Autodesk Inventor part; units mm, degrees
ref_plane "YZ Plane" through (0, 0, 0) normal (1, 0, 0) x (0, 1, 0)
ref_plane "XZ Plane" through (0, 0, 0) normal (0, 1, 0) x (-1, 0, 0)
ref_plane "XY Plane" through (0, 0, 0) normal (0, 0, 1) x (1, 0, 0)
sketch "Sketch1" plane through (0, 0, 0) normal (0, 1, 0) x (-1, 0, 0)
  line L0 (32.355, 4.45) -> (-32.355, 4.45)
  line L1 (-32.355, 4.45) -> (-32.355, -4.45)
  line L2 (-32.355, -4.45) -> (32.355, -4.45)
  line L3 (32.355, -4.45) -> (32.355, 4.45)
  point P0 (0, 0)
  dimension "d0" = 64.71
  dimension "d1" = 32.355
  dimension "d2" = 8.9
  dimension "d3" = 4.45
extrude "Extrusion1" add sketch "Sketch1" along normal blind 7.8
sketch "Sketch2" plane through (0, 0, 0) normal (0, 1, 0) x (-1, 0, 0)
  line L0 (-32.355, 4.45) -> (-32.355, -4.45)
  line L1 (-32.355, -3.45) -> (-37.945, -3.45)
  line L2 (-37.945, -3.45) -> (-37.945, 6.25)
  line L3 (-37.945, 6.25) -> (-32.355, 6.25)
  line L4 (-32.355, 6.25) -> (-32.355, -3.45)
  line L5 (-32.355, -4.45) -> (32.355, -4.45)
  line L6 (32.355, -4.45) -> (32.355, 4.45)
  line L7 (32.355, -3.45) -> (37.855, -3.45)
  line L8 (37.855, -3.45) -> (37.855, 6.25)
  line L9 (37.855, 6.25) -> (32.355, 6.25)
  line L10 (32.355, 6.25) -> (32.355, -3.45)
  point P0 (0, 0)
  dimension "d6" = 10.7
  dimension "d7" = 5.59
  dimension "d8" = 10.7
  dimension "d9" = 5.5
  dimension "d10" = 1
  dimension "d11" = 1
extrude "Extrusion2" add sketch "Sketch2" along normal blind 5
sketch "Sketch3" plane through (-32.355, 7.8, 4.45) normal (0, 0, 1) x (1, 0, 0)
  line L0 (0, -2.8) -> (0, 0)
  line L1 (64.71, -7.8) -> (64.71, 0)
  line L2 (0, -2.8) -> (64.71, -2.8)
  line L3 (64.71, -2.8) -> (64.71, -1.35)
  line L4 (64.71, -1.35) -> (0, -1.35)
  line L5 (0, -1.35) -> (0, -2.8)
  point P0 (32.355, -7.8)
  dimension "d14" = 1.45
extrude "Extrusion3" cut sketch "Sketch3" against normal blind 5
sketch "Sketch4" plane through (0, 5, 0) normal (0, 1, 0) x (1, 0, 0)
  line L0 (32.355, -6.25) -> (37.945, -6.25)
  line L1 (37.945, 3.45) -> (32.355, 3.45)
  line L2 (37.945, -6.25) -> (32.355, -6.25)
  line L3 (32.355, -6.25) -> (32.355, 3.45)
  line L4 (32.355, 3.45) -> (37.945, 3.45)
  line L5 (37.945, 3.45) -> (37.945, -6.25)
  line L6 (-37.855, -6.25) -> (-32.355, -6.25)
  line L7 (-32.355, 3.45) -> (-37.855, 3.45)
  line L8 (-37.855, -6.25) -> (-32.355, -6.25)
  line L9 (-32.355, -6.25) -> (-32.355, 3.45)
  line L10 (-32.355, 3.45) -> (-37.855, 3.45)
  line L11 (-37.855, 3.45) -> (-37.855, -6.25)
  line L12 (-37.355, -5.75) -> (-32.855, -5.75)
  line L13 (-32.855, -5.75) -> (-32.855, 2.95)
  line L14 (-32.855, 2.95) -> (-37.355, 2.95)
  line L15 (-37.355, 2.95) -> (-37.355, -5.75)
  line L16 (32.855, -5.75) -> (37.445, -5.75)
  line L17 (37.445, -5.75) -> (37.445, 2.95)
  line L18 (37.445, 2.95) -> (32.855, 2.95)
  line L19 (32.855, 2.95) -> (32.855, -5.75)
  point P0 (0, 0)
  dimension "d17" = 0.5
  dimension "d18" = 0.5
extrude "Extrusion4" add sketch "Sketch4" along normal blind 0.5 contours L15 L14 L13 L12 | L19 L18 L17 L16
sketch "Sketch5" plane through (0, 5.5, 0) normal (0, 1, 0) x (1, 0, 0)
  circle A0 centre (35.205, -4.05) radius 1.15
  circle A1 centre (-35.205, -4.1) radius 1.15
  point P0 (0, 0)
  dimension "d21" = 4.1
  dimension "d22" = 4.05
  dimension "d23" = 70.41
  dimension "d24" = 35.205
  dimension "d35" = 2.3
  dimension "d36" = 2.3
extrude "Extrusion5" cut sketch "Sketch5" against normal through all
sketch "Sketch6" plane through (0, 0, 0) normal (0, -1, 0) x (1, 0, 0)
  circle A0 centre (30.75, 0) radius 0.75
  circle A1 centre (-30.75, 0) radius 0.75
  point P0 (0, 0)
  dimension "d27" = 61.5
  dimension "d28" = 30.75
  dimension "d29" = 1.5
  dimension "d30" = 1.5
  dimension "d33" = 0
  dimension "d34" = 0
extrude "Extrusion6" add sketch "Sketch6" along normal blind 1
sketch "Sketch7" plane through (-32.355, 0, 4.45) normal (0, 0, 1) x (1, 0, 0)
  line L0 (64.71, 0) -> (0, 0)
  line L1 (7.805, 0) -> (8.805, 0)
  line L2 (8.805, 0) -> (8.805, 7.7141)
  line L3 (8.805, 7.7141) -> (7.805, 7.7141)
  line L4 (7.805, 7.7141) -> (7.805, 0)
  point P0 (32.355, 0)
  dimension "d37" = 1
  dimension "d38" = 23.55
extrude "Extrusion7" add sketch "Sketch7" along normal mid plane 1
properties part number "QSevenConnector"
Can you work these out from the model? Positions are in its coordinate system, mm. A direction names the side the tool comes from. Give positions to 0.01 mm unless a question says otherwise; leave off trailing zeros. Order: outer loops, then holes, each group sorted by start corner. A loop starts at its lowest first (then second) coordinate and runs counter-clockwise, first axis right, second up. Notation, with made-up numbers: M 15,54.5 L 46,54.5 A37 cw 46,90.5 Z; hole C 19.25,-36.5 d3. An arc over 180 degrees is marked long. Use a Markdown table: item, result. Add a question column.
Item 1: Suppose I cut it at C-C (x = 30.75). List the corners of the cut face in (y, z) for me, then the cut area to 3 significant figures.
Item 2: Suppose I cut it at A-A (x = -16.5). List the corners of the cut face in (y, z) for me.
Item 3: For faces 4 (the flat face through (35, 2, -3.45)), 5 (the cylindrical face through (31.465, -0.493, -0.225)), 6 (the flat face through (-35, 2, -3.45)), 7 (the flat face through (-29, 2, 4.45)), 8 (the flat face through (-35, 5.5, 1)), which set-ups out of +Z, -Z, +X, -X, +Y, -Y let a thin tool reach every point of the face, with its end or its side?
Item 4: If I drill on L1, parallel to X at y = 1.4, z = 4.1 (3 decimals); L2, parallel to Y at x = 12.5, z = 4.25; L3, parallel to X at y = 3, z = 4.5 (3 decimals), over which ranges is the centre line in solid material (lowest first)? Write a range as [from, to].
Item 5: Suppose I cut it at B-B (y = 3). List the corners of the cut face in (x, z) for me (3 decimals), then the cut area to 3 significant figures.
Item 6: We'd pull the mould along X, two halves only. Please class faces 1 (the flat face through (0, 6.45, 2)), 2 (the flat face through (4, 2, 4.45)), 3 (the flat face through (37.945, 2, 1)): +X half, -X half, draft (parallel to the pull), parting line (faces both ways), or undercut.
Item 7: Will these pins go through, and if not, where does the flat tip stop? pin 1 (3.5 mm diameter, centred on x = -35.205, z = 4.1, fed in from +Y); pin 2 (3 mm diameter, centred on x = -12.5, z = 2.5, fed in from -Y); pin 3 (0.7 mm diameter, centred on x = 9, y = 5.5, fed in from +Z).
Answer sheet:
| question | item | result |
|---|---|---|
| 1 | outline | M -1,-0.75 L 0,-0.75 L 0,-4.45 L 7.8,-4.45 L 7.8,4.45 L 6.45,4.45 L 6.45,-0.55 L 5,-0.55 L 5,4.45 L 0,4.45 L 0,0.75 L -1,0.75 Z |
| 1 | area | 63.7 mm² |
| 2 | outline | M 0,-4.45 L 7.8,-4.45 L 7.8,4.45 L 6.45,4.45 L 6.45,-0.55 L 5,-0.55 L 5,4.45 L 0,4.45 Z |
| 3 | face 4 | -Z, +X, +Y, -Y |
| 3 | face 5 | -Y |
| 3 | face 6 | -Z, -X, +Y, -Y |
| 3 | face 7 | +Z, +Y, -Y |
| 3 | face 8 | +Z, -Z, -X, +Y |
| 4 | L1 | x = [-37.855, -36.355], [-34.055, 34.056], [36.354, 37.945] |
| 4 | L2 | y = [0, 5], [6.45, 7.8] |
| 4 | L3 | x = [-37.855, -36.283], [-34.127, -32.355], [-24.55, -23.55], [32.355, 34.147], [36.263, 37.945] |
| 5 | outline | M -37.855,-3.45 L -32.355,-3.45 L -32.355,-4.45 L 32.355,-4.45 L 32.355,-3.45 L 37.945,-3.45 L 37.945,6.25 L 32.355,6.25 L 32.355,4.45 L -23.55,4.45 L -23.55,4.95 L -24.55,4.95 L -24.55,4.45 L -32.355,4.45 L -32.355,6.25 L -37.855,6.25 Z; hole C -35.205,4.1 d2.3; hole C 35.205,4.05 d2.3 |
| 5 | area | 676 mm² |
| 6 | face 1 | draft |
| 6 | face 2 | undercut |
| 6 | face 3 | +X half |
| 7 | pin 1 | stops at y = 5.5 |
| 7 | pin 2 | stops at y = 0 |
| 7 | pin 3 | stops at z = -0.55 |
